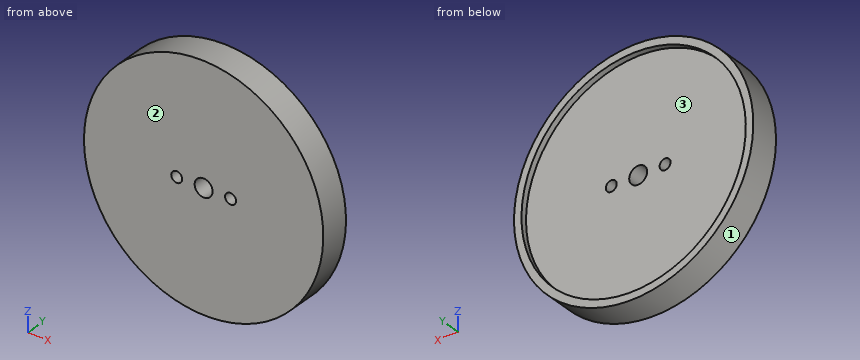
from build123d import *

# Parameters (mm, degrees)
SKETCH2_R           = 40
SKETCH2_R_2         = 37.5
BOSS_EXTRUDE1_DEPTH = 10
SKETCH2_4_R         = 37.5
SKETCH2_4_R_2       = 1.835
SKETCH2_4_R_3       = 3
BOSS_EXTRUDE2_DEPTH = 8


with BuildPart() as part:
    # Sketch2 → Boss-Extrude1 (new body)
    with BuildSketch(Plane(origin=(0, 0, 0), x_dir=(1, 0, 0), z_dir=(0, 1, 0))):
        with Locations(Location((0, 0, 0), (0, 0, 270))):
            Circle(SKETCH2_R)
        with Locations(Location((0, 0, 0), (0, 0, 270))):
            Circle(SKETCH2_R_2, mode=Mode.SUBTRACT)
    extrude(amount=BOSS_EXTRUDE1_DEPTH)

    # Sketch2_4 → Boss-Extrude2 (add)
    with BuildSketch(Plane(origin=(0, 0, 0), x_dir=(1, 0, 0), z_dir=(0, 1, 0))):
        with Locations(Location((0, 0, 0), (0, 0, 270))):
            Circle(SKETCH2_4_R)
        with Locations(Location((-9, 0, 0), (0, 0, 270))):
            Circle(SKETCH2_4_R_2, mode=Mode.SUBTRACT)
        with Locations(Location((9, 0, 0), (0, 0, 270))):
            Circle(SKETCH2_4_R_2, mode=Mode.SUBTRACT)
        with Locations(Location((0, 0, 0), (0, 0, 270))):
            Circle(SKETCH2_4_R_3, mode=Mode.SUBTRACT)
    extrude(amount=BOSS_EXTRUDE2_DEPTH)


solid = part.part
Could you check a few things on this model? Use its own coordinates, in mm. Face numbers are marked on the shaded views. Coordinates: 2 decimals unless noted, no trailing zeros. Write each loop counter-clockwise with the first axis right and the second up, starting at its lowest first coordinate (ties: lowest second). Pieces come first, ordered by that corner, then holes. Notation, with made-up numbers: (-3.5, -33) - (22.5, -33) arc R13 ccw to (22.5, -25) - close; hole circle Ø2 at (43, 10). An arc over 180 degrees is marked (long way). Write item = value, one per line.
1) Please list where these lines run through material, in increasing order: line 1 (X direction, y = 5, z = 0) (3 decimals); line 2 (Z direction, x = 10, y = 3.75); line 3 (Y direction, x = 9.5, z = 11.5). Write a range as [from, to].
Result set:
line_1 = [-40, -10.835], [-7.165, -3], [3, 7.165], [10.835, 40]
line_2 = [-38.73, -1.54], [1.54, 38.73]
line_3 = [0, 8]
2) Suppose I cut it at B-B on x = 0. Please give me the cut outline in (y, z), plus the area to 3 significant figures.
Result set:
outline = (0, -40) - (10, -40) - (10, -37.5) - (8, -37.5) - (8, -3) - (0, -3) - close; (0, 3) - (8, 3) - (8, 37.5) - (10, 37.5) - (10, 40) - (0, 40) - close
area = 602 mm2
3) Suppose I cut it at C-C on y = 7. Please give me the cut outline in (x, z) (3 decimals), plus the area to 3 significant figures.
Result set:
outline = circle Ø80 at (0, 0); hole circle Ø3.67 at (-9, 0); hole circle Ø6 at (0, 0); hole circle Ø3.67 at (9, 0)
area = 4,980 mm2
4) We'd pull the mould along X, two halves only. Please class the marked faces 1, 2 and 3: +X half, -X half, draft (parallel to the pull), parting line (faces both ways), or undercut.
Result set:
face_1 = parting line
face_2 = draft
face_3 = undercut
5) Suppose I cut it at A-A on z = 0. Please give me the cut outline in (x, y) (3 decimals).
Result set:
outline = (-40, 0) - (-10.835, 0) - (-10.835, 8) - (-37.5, 8) - (-37.5, 10) - (-40, 10) - close; (-7.165, 0) - (-3, 0) - (-3, 8) - (-7.165, 8) - close; (3, 0) - (7.165, 0) - (7.165, 8) - (3, 8) - close; (10.835, 0) - (40, 0) - (40, 10) - (37.5, 10) - (37.5, 8) - (10.835, 8) - close
6) Suppose I cut it at D-D on z = 32.5. Please give me the cut outline in (x, y).
Result set:
outline = (-23.32, 0) - (23.32, 0) - (23.32, 10) - (18.71, 10) - (18.71, 8) - (-18.71, 8) - (-18.71, 10) - (-23.32, 10) - close
7) Will these pins go through, and if not, where does the flat tip stop? pin 1 Ø5 at (x, z) = (-9, 0) entering from +Y; pin 2 Ø6 at (y, z) = (2.5, 14.5) entering from -X; pin 3 Ø4 at (y, z) = (5.5, -17.5) entering from +X; pin 4 Ø2 at (x, z) = (9, 0) entering from +Y (3 decimals).
Result set:
pin_1 = 8
pin_2 = -38.31
pin_3 = 36.87
pin_4 = through
